The model under review builds one solid part; all positions refer to its coordinate system, in mm. A direction names the side the tool comes from. Coordinates: 2 decimals unless noted, no trailing zeros. Write each loop counter-clockwise with the first axis right and the second up, starting at its lowest first coordinate (ties: lowest second). Pieces come first, ordered by that corner, then holes. Notation, with made-up numbers: (7, -9) -> (63, -9) arc R18 cw to (63, -2) -> close; hole circle Ø4 at (62, 59.25). An arc over 180 degrees is marked (long way). Write each question's results on one line, items separated by ' | '.
```python
from build123d import *

# Parameters (mm, degrees)
F0_R     = 22.225
F0_R_2   = 11.1125
F1_DEPTH = 23.1302697212


# Not quite as in the source:
# - a feature of the source that left no trace in its solid (it failed there, or was rolled back) is left out


with BuildPart() as f1:
    # F0 (on Front) → F1 (new body)
    with BuildSketch(Plane.XZ):
        with BuildLine():
            ThreePointArc((3.175, 31.5908511281), (23.5464301965, 21.2985474857), (31.75, 0))
            ThreePointArc((31.75, 0), (23.5464301965, -21.2985474857), (3.175, -31.5908511281))
            Line((3.175, -31.5908511281), (160.3375, -15.7954255641))
            ThreePointArc((160.3375, -15.7954255641), (142.875, 0), (160.3375, 15.7954255641))
            Line((160.3375, 15.7954255641), (3.175, 31.5908511281))
        make_face()
        with BuildLine():
            ThreePointArc((42.9352789855, -11.5049692931), (44.4472073469, 0.4982560178), (42.6665789099, 12.4645715579))
            ThreePointArc((42.6665789099, 12.4645715579), (43.8780302599, 18.3037033525), (49.3968044685, 20.5633948632))
            Line((49.3968044685, 20.5633948632), (121.9253365113, 13.2740031244))
            ThreePointArc((121.9253365113, 13.2740031244), (126.3702809224, 10.7659070162), (127.5336137594, 5.7965274156))
            ThreePointArc((127.5336137594, 5.7965274156), (127.0030897981, 0.4429363765), (127.3840485491, -4.9233717695))
            ThreePointArc((127.3840485491, -4.9233717695), (126.1371549085, -9.7886185026), (121.7458582589, -12.226216349))
            Line((121.7458582589, -12.226216349), (49.7038902692, -19.4667065606))
            ThreePointArc((49.7038902692, -19.4667065606), (44.2309158386, -17.261504048), (42.9352789855, -11.5049692931))
        make_face(mode=Mode.SUBTRACT)
        with BuildLine():
            ThreePointArc((3.175, -31.5908511281), (23.5464301965, -21.2985474857), (31.75, 0))
            ThreePointArc((31.75, 0), (23.5464301965, 21.2985474857), (3.175, 31.5908511281))
            ThreePointArc((3.175, 31.5908511281), (-31.75, 0), (3.175, -31.5908511281))
        make_face()
        Circle(F0_R, mode=Mode.SUBTRACT)
        with BuildLine():
            ThreePointArc((174.625, 0), (170.5232150983, 10.6492737428), (160.3375, 15.7954255641))
            ThreePointArc((160.3375, 15.7954255641), (142.875, 0), (160.3375, -15.7954255641))
            ThreePointArc((160.3375, -15.7954255641), (170.5232150983, -10.6492737428), (174.625, 0))
        make_face()
        with Locations((158.75, 0)):
            Circle(F0_R_2, mode=Mode.SUBTRACT)
    extrude(amount=F1_DEPTH)


solid = f1.part
```
Q1. Add section D-D (x = 78). Write out the cut boundary in (y, z).
Solution:
outline: (-23.13, -24.07) -> (0, -24.07) -> (0, -16.62) -> (-23.13, -16.62) -> close; (-23.13, 17.69) -> (0, 17.69) -> (0, 24.07) -> (-23.13, 24.07) -> close
Q2. Machinability: for faces 1 (the cylindrical face through (44.29, -11.4, -17.33)), 2 (the flat face through (80.7, -11.4, -23.8)), which of the approach directions +Z, -Z, +X, -X, +Y, -Y give a long, thin tool a straight path to every point of the face, cutting with its end or side? Answer none if there is none.
Solution:
face 1: +Y, -Y | face 2: -Z, +X, +Y, -Y
Q3. Clearance check with flat-ended pins moving along their axes: P1, Ø1.5, axis at x = 42, y = -8.5, coming from the +Z side; P2, Ø2, axis at x = 78.5, y = -20.5, coming from the -Z side; P3, Ø6, axis at x = 87, y = -20, coming from the +Z side. State where each tip first meets the part, or that it passes through.
Solution:
P1: z = 27.76 | P2: z = -24.12 | P3: z = 23.47
Q4. For line 1 (X direction, y = -13, z = 5); line 2 (X direction, y = -6.5, z = -5.5); line 3 (Z direction, x = -15, y = -14.25), list the stretches that pass through material, from the lowest coordinate up. Write a range as from..to.
Solution:
line 1: -31.35..-21.66, 21.66..44.17, 127.4..148.83, 168.67..173.82 | line 2: -31.27..-21.53, 21.53..44.11, 127.45..149.09, 168.41..173.64 | line 3: -27.98..-16.4, 16.4..27.98
Q5. Add section C-C (y = -13). Count the separate pieces of the cut face and the enclosed holes in it, plus the area to 3 significant figures.
Solution:
separate pieces: 1 | enclosed holes: 3 | area: 4,910 mm²
Q6. Add section A-A (x = 0). Write out the cut boundary in (y, z) (3 decimals).
Solution:
outline: (-23.13, -31.75) -> (0, -31.75) -> (0, -22.225) -> (-23.13, -22.225) -> close; (-23.13, 22.225) -> (0, 22.225) -> (0, 31.75) -> (-23.13, 31.75) -> close
Q7. Add section B-B (z = -2.5). Write out the cut boundary in (x, y), plus the area to 3 significant figures.
Solution:
outline: (-31.65, -23.13) -> (-22.08, -23.13) -> (-22.08, 0) -> (-31.65, 0) -> close; (22.08, -23.13) -> (44.38, -23.13) -> (44.38, 0) -> (22.08, 0) -> close; (127.1, -23.13) -> (147.92, -23.13) -> (147.92, 0) -> (127.1, 0) -> close; (169.58, -23.13) -> (174.43, -23.13) -> (174.43, 0) -> (169.58, 0) -> close | area: 1,330 mm²
Q8. Draft analysis for pull direction Z (two halves, no side actions). For faces 3 (the flat face through (82.856, -11.403, 23.583)), 4 (the cylindrical face through (-31.74, -11.4, 0.74)), 5 (the flat face through (86.2, -11.4, -15.8)), 6 (the cylindrical face through (126.18, -11.4, -9.73)), state which applies: pulls with the +Z half, pulls with the -Z half, needs draft (parallel to the pull), parting line crosses it, or undercut.
Solution:
face 3: pulls with the +Z half | face 4: parting line crosses it | face 5: undercut | face 6: undercut
